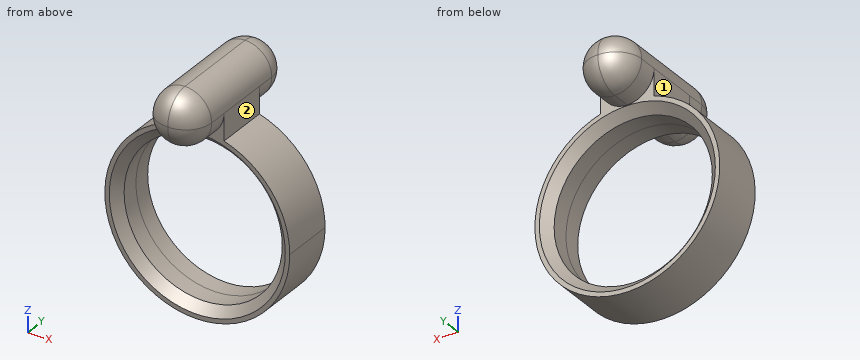
from build123d import *

# Parameters (mm, degrees)
F0_R          = 8.875
F1_DEPTH      = 3
F1_DEPTH_BACK = 3
F2_SIZE       = 1
F3_DEPTH      = 8
F3_DEPTH_BACK = 8
F4_R          = 2.99999
F5_R          = 2.9


# Not quite as in the source:
# - a fillet or chamfer is up to 0.001 mm smaller than in the source, because OpenCascade refuses the exact size
# - a feature names something its author has since deleted; it is built from what else it names


with BuildPart() as f1:
    # F0 (on Front) → F1 (new body, two sides)
    with BuildSketch(Plane.XZ) as f1_sk:
        with BuildLine():
            ThreePointArc((-3, 9.931798679), (-6.1852900094, -8.3296345958), (10.375, 0))
            ThreePointArc((10.375, 0), (8.3296345958, 6.1852900094), (3, 9.931798679))
            Line((3, 9.931798679), (-3, 9.931798679))
        make_face()
        Circle(F0_R, mode=Mode.SUBTRACT)
    extrude(amount=F1_DEPTH)
    extrude(f1_sk.sketch, amount=-F1_DEPTH_BACK)

    # F2
    f2_edges = [f1.edges().sort_by_distance(p)[0] for p in [
        (-8.875, -3, 0),
        (-8.875, 3, 0),
    ]]
    chamfer(f2_edges, length=F2_SIZE)

    # F0 (on Front) → F3 (join, two sides)
    with BuildSketch(Plane.XZ) as f3_sk:
        with BuildLine():
            ThreePointArc((-3, 9.931798679), (0, 10.375), (3, 9.931798679))
            Line((3, 9.931798679), (3, 15.931798679))
            Line((3, 15.931798679), (-3, 15.931798679))
            Line((-3, 15.931798679), (-3, 9.931798679))
        make_face()
        with BuildLine():
            Line((-3, 9.931798679), (3, 9.931798679))
            ThreePointArc((3, 9.931798679), (0, 10.375), (-3, 9.931798679))
        make_face()
    extrude(amount=F3_DEPTH)
    extrude(f3_sk.sketch, amount=-F3_DEPTH_BACK)

    # F4 (radius 3 in the source; OpenCascade refuses exactly that, so slightly less here)
    f4_edges = [f1.edges().sort_by_distance(p)[0] for p in [
        (-3, 0, 15.931799),
        (3, 0, 15.931799),
        (3, -5.5, 9.931799),
        (3, 5.5, 9.931799),
        (-3, -5.5, 9.931799),
        (-3, 5.5, 9.931799),
    ]]
    fillet(f4_edges, radius=F4_R)

    # F5
    f5_edges = [f1.edges().sort_by_distance(p)[0] for p in [
        (2.121323, -8, 15.053122),
        (2.121323, 8, 15.053122),
        (3, -8, 12.931799),
        (3, 8, 12.931799),
        (2.121323, -8, 10.810475),
        (0, -8, 9.931799),
        (0, -8, 15.931799),
        (-2.121323, -8, 10.810475),
        (-2.121323, -8, 15.053122),
        (-3, -8, 12.931799),
        (2.121323, 8, 10.810475),
        (0, 8, 9.931799),
        (0, 8, 15.931799),
        (-2.121323, 8, 10.810475),
        (-2.121323, 8, 15.053122),
        (-3, 8, 12.931799),
    ]]
    fillet(f5_edges, radius=F5_R)


solid = f1.part
Design review of the part built by this model. Coordinates are the model's own, in mm. Face numbers are marked on the shaded views. A direction names the side the tool comes from. Round coordinates to 2 decimals unless told otherwise and drop trailing zeros.
Item 1: For pin 1 Ø8 at (x, y) = (5.5, -3) entering from -Z; pin 2 Ø10.5 at (x, z) = (0, 0) entering from +Y; pin 3 Ø5 at (x, z) = (-7.5, -7.5) entering from -Y; pin 4 Ø1 at (x, y) = (1, -4) entering from +Z, all flat-tipped, find the tip position at first contact; note any pin that passes through.
Item 2: For the marked faces 1 and 2, list the 3-axis set-ups (+Z, -Z, +X, -X, +Y, -Y) from which the entire face can be reached by the end or side of a thin tool; tool diameter is ignored.
Item 3: Wall thickness on L1, parallel to Z at x = 0, y = 1.3 (3 decimals); L2, parallel to Z at x = 1.5, y = -1.5; L3, parallel to X at y = 1, z = -6.25: over which ranges is each line inside the solid? List them lowest first.
Check values:
1. pin 1: stops at z = -10.27
1. pin 2: passes through
1. pin 3: stops at y = -3
1. pin 4: stops at z = 15.89
2. face 1: +Z, -X, +Y, -Y
2. face 2: +Z, +X, +Y, -Y
3. L1: z = -10.375 to -8.875, 8.875 to 15.932
3. L2: z = -10.27 to -8.75, 8.75 to 15.53
3. L3: x = -8.28 to -6.3, 6.3 to 8.28
